from build123d import *

# Parameters (mm, degrees)
PAD_DEPTH    = 31.75
SKETCH001_R  = 3.175
SKETCH001_W  = 2.54
SKETCH001_H  = 12.7
POCKET_DEPTH = 12.701


with BuildPart() as part:
    # Sketch → Pad (new body)
    with BuildSketch(Plane.XY):
        with BuildLine():
            Line((0, 51.181), (12.7, 51.181))
            Line((12.7, 51.181), (12.7, 25.781))
            ThreePointArc((0, -28.739345), (27.989989, -6.520004), (12.7, 25.781))
            Line((0, -19.431), (0, -28.739345))
            ThreePointArc((0, -19.431), (19.431, 0), (0, 19.431))
            Line((0, 51.181), (0, 19.431))
        make_face()
    extrude(amount=PAD_DEPTH)

    # Sketch001 (on Face2 of Pad) → Pocket (cut, through all)
    with BuildSketch(Plane.YZ.offset(12.7)):
        with Locations((38.481, 7.62)):
            Circle(SKETCH001_R)
        with Locations((27.051, 21.59)):
            Rectangle(SKETCH001_W, SKETCH001_H)
    extrude(amount=-POCKET_DEPTH, mode=Mode.SUBTRACT)


solid = part.part
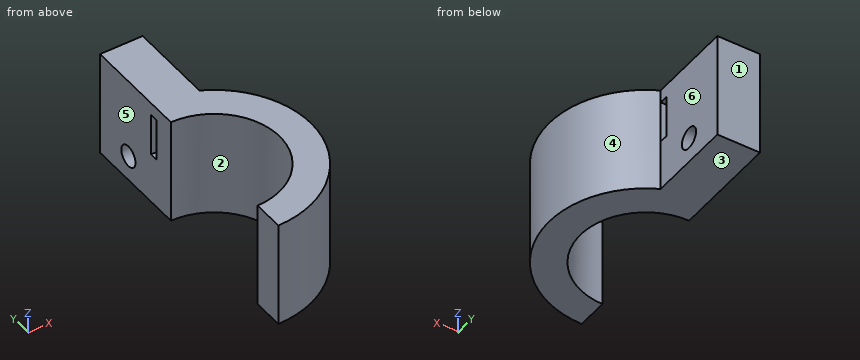
Read the model definition and answer for the solid it produces. Units are mm, in the model's axes. Face numbers are marked on the shaded views. A direction names the side the tool comes from. Round coordinates to 2 decimals unless told otherwise and drop trailing zeros. Write each loop counter-clockwise with the first axis right and the second up, starting at its lowest first coordinate (ties: lowest second). Pieces come first, ordered by that corner, then holes.
1. Given pin 1 Ø1.5 at (x, z) = (10.5, 4.5) entering from -Y; pin 2 Ø12 at (y, z) = (23.5, 25) entering from +X; pin 3 Ø7.5 at (y, z) = (41.5, 22) entering from +X, each flat-ended and moving along its own axis, determine where each tip first touches the part or whether it passes through.
2. The part is cut by section D-D, the plane y = 0. Determine the outline of the cut face in (x, z), then the cut area to 3 significant figures.
3. The part is cut by section A-A, the plane z = 22. Determine the outline of the cut face in (x, y).
4. The part is cut by section C-C, the plane z = 7.62. Determine the outline of the cut face in (x, y).
5. Determine the mould class of the marked faces 1, 2, 3 and 4 for opening direction Y: pulls with the +Y half, pulls with the -Y half, needs draft (parallel to the pull), parting line crosses it, or undercut.
6. Straight lines are drawn through the part: L1, parallel to Y at x = 7.5, z = 13; L2, parallel to Z at x = 11.5, y = 38; L3, parallel to X at y = 47.5, z = 12. For each, find the intervals that lie inside material, in ascending order.
7. The part is cut by section B-B, the plane x = 6. Determine the outline of the cut face in (y, z) (3 decimals), then the cut area to 3 significant figures.
8. Which of the six approach directions +Z, -Z, +X, -X, +Y, -Y give full straight-line access (tool end or side, diameter ignored) to the marked faces 5 and 6?
Values:
1. pin 1: stops at y = -27.03
1. pin 2: stops at x = 22.8
1. pin 3: stops at x = 12.7
2. outline: (19.43, 0) - (28.74, 0) - (28.74, 31.75) - (19.43, 31.75) - close
2. area: 296 mm2
3. outline: (0, -28.74) arc R28.74 ccw to (12.7, 25.78) - (0, 25.78) - (0, 19.43) arc R19.43 cw to (0, -19.43) - close; (0, 28.32) - (12.7, 28.32) - (12.7, 51.18) - (0, 51.18) - close
4. outline: (0, -28.74) arc R28.74 ccw to (12.7, 25.78) - (12.7, 35.31) - (0, 35.31) - (0, 19.43) arc R19.43 cw to (0, -19.43) - close; (0, 41.66) - (12.7, 41.66) - (12.7, 51.18) - (0, 51.18) - close
5. face 1: pulls with the +Y half
5. face 2: undercut
5. face 3: needs draft
5. face 4: parting line crosses it
6. L1: y = -27.74 to -17.93, 17.93 to 51.18
6. L2: z = 0 to 4.48, 10.76 to 31.75
6. L3: x = 0 to 12.7
7. outline: (-28.106, 0) - (-18.481, 0) - (-18.481, 31.75) - (-28.106, 31.75) - close; (18.481, 0) - (51.181, 0) - (51.181, 31.75) - (18.481, 31.75) - close; hole (25.781, 15.24) - (28.321, 15.24) - (28.321, 27.94) - (25.781, 27.94) - close; hole circle Ø6.35 at (38.481, 7.62)
7. area: 1,280 mm2
8. face 5: +Z, -Z, -X, +Y, -Y
8. face 6: +Z, -Z, +X, +Y
